from build123d import *

# Parameters (mm, degrees)
SKETCH1_R           = 42.5
BOSS_EXTRUDE1_DEPTH = 75
SKETCH2_R           = 27.5
BOSS_EXTRUDE2_DEPTH = 40
CUT_EXTRUDE1_DEPTH  = 130.759392724


with BuildPart() as part:
    # Sketch1 → Boss-Extrude1 (new, symmetric)
    with BuildSketch(Plane(origin=(0, 0, 0), x_dir=(-1, 0, 0), z_dir=(0, 1, 0))):
        with Locations(Location((0, 0, 0), (0, 0, 90))):
            Circle(SKETCH1_R)
    extrude(amount=BOSS_EXTRUDE1_DEPTH, both=True)

    # Sketch2 → Boss-Extrude2 (add)
    with BuildSketch(Plane(origin=(0, 75, 0), x_dir=(-1, 0, 0), z_dir=(0, 1, 0))):
        with Locations(Location((0, 0, 0), (0, 0, 90))):
            Circle(SKETCH2_R)
    boss_extrude2 = extrude(amount=BOSS_EXTRUDE2_DEPTH)

    # Sketch3 → Cut-Extrude1 (cut, symmetric)
    with BuildSketch(Plane.YZ):
        Polygon((91, 27.5), (91, 19.5), (101.5, 19.5), (101.5, 27.5), (101.5, 29.5), (91, 29.5), align=None)
    cut_extrude1 = extrude(amount=CUT_EXTRUDE1_DEPTH, both=True, mode=Mode.SUBTRACT)

    # Mirror1: Boss-Extrude2, Cut-Extrude1 across plane
    add(boss_extrude2.mirror(Plane.ZX))
    add(cut_extrude1.mirror(Plane.ZX), mode=Mode.SUBTRACT)


solid = part.part
Geometry: final body of the model. Coordinates: model frame, mm. A direction names the side the tool comes from. Round coordinates to 2 decimals unless told otherwise and drop trailing zeros. Loops run counter-clockwise (first coordinate to the right, second up) from the corner with the lowest first, then second, coordinate; pieces in that order, holes last.
Q1. Pin query (flat end, axial travel): P1, Ø1.5, axis at x = 23, z = 17, coming from the +Y side; P2, Ø1.5, axis at x = -32.5, y = 42, coming from the -Z side; P3, Ø5, axis at y = -50, z = -1.5, coming from the -X side. Return the tip coordinate at first contact, or that it passes through.
Q2. Pull-direction query (Y, two-part tool) for faces 5 (the cylindrical face through (-25.861, 1.05, -33.727)), 6 (the flat face through (0, 115, 0)), 7 (the flat face through (0, 101.5, 23)); classes: released by +Y, released by -Y, zero draft, split by the parting line, or undercut.
Q3. Material intervals for L1, parallel to X at y = -58, z = -2; L2, parallel to Y at x = 16, z = -31; L3, parallel to Z at x = -20, y = -47.5, sorted ascending.
Q4. Access query for faces 1 (the flat face through (0, 96, 19.5)), 2 (the flat face through (1, -75, 28)), 3 (the flat face through (0, -115, 0)), 4 (the cylindrical face through (1.209, 94.72, -27.473)). Directions: +Z, -Z, +X, -X, +Y, -Y. A direction counts if a zero-diameter tool reaches every point of the face in a straight line with its end or side. Return the directions, or none.
Q5. Section C-C on y = -49. Return loops of the section in (x, z).
Q6. Section A-A on x = 0. Return loops of the section in (y, z).
Q7. Section B-B on z = 0. Return loops of the section in (x, y), plus the area to 4 significant figures.
Q8. Section D-D on x = -25. Return loops of the section in (y, z), plus the area to 3 significant figures.
Evaluation:
1. P1: stops at y = 75
1. P2: stops at z = -28.25
1. P3: stops at x = -42.5
2. face 5: zero draft
2. face 6: released by +Y
2. face 7: undercut
3. L1: x = -42.45 to 42.45
3. L2: y = -75 to 75
3. L3: z = -37.5 to 37.5
4. face 1: +Z, +X, -X
4. face 2: -Y
4. face 3: +Z, -Z, +X, -X, -Y
4. face 4: +Y
5. outline: circle Ø85 at (0, 0)
6. outline: (-115, -27.5) - (-75, -27.5) - (-75, -42.5) - (75, -42.5) - (75, -27.5) - (115, -27.5) - (115, 27.5) - (101.5, 27.5) - (101.5, 19.5) - (91, 19.5) - (91, 27.5) - (75, 27.5) - (75, 42.5) - (-75, 42.5) - (-75, 27.5) - (-91, 27.5) - (-91, 19.5) - (-101.5, 19.5) - (-101.5, 27.5) - (-115, 27.5) - close
7. outline: (-42.5, -75) - (-27.5, -75) - (-27.5, -115) - (27.5, -115) - (27.5, -75) - (42.5, -75) - (42.5, 75) - (27.5, 75) - (27.5, 115) - (-27.5, 115) - (-27.5, 75) - (-42.5, 75) - close
7. area: 17,150 mm2
8. outline: (-115, -11.46) - (-75, -11.46) - (-75, -34.37) - (75, -34.37) - (75, -11.46) - (115, -11.46) - (115, 11.46) - (75, 11.46) - (75, 34.37) - (-75, 34.37) - (-75, 11.46) - (-115, 11.46) - close
8. area: 12,100 mm2
